from build123d import *

# Parameters (mm, degrees)
F3_W     = 10
F3_H     = 5
F8_DEPTH = 10
F9_T     = -1


with BuildPart() as f6:
    # F6: sweep along a path in F5
    with BuildLine(Plane(origin=(0, 0, 0), x_dir=(0.5735764364, 0.8191520443, 0), z_dir=(0.8191520443, -0.5735764364, 0))) as f6_path:
        Line((-28.3761330307, -7.5), (-32.7062600496, -5))
    # F3 (on line) → F6 (sweep)
    with BuildSketch(Plane(origin=(-18.7595400856, -26.7913997807, 0), x_dir=(-0.8191520443, 0.5735764364, 0), z_dir=(0.5735764364, 0.8191520443, 0))):
        with Locations((0, -5)):
            Rectangle(F3_W, F3_H)
    sweep(path=f6_path.line)

    # F7 (on face) → F8 (cut, through all)
    with BuildSketch(Plane(origin=(4.0957602214, -2.8678821818, 0), x_dir=(0.5735764364, 0.8191520443, 0), z_dir=(0.8191520443, -0.5735764364, 0))):
        Polygon((-28.3761330307, -10), (-28.3761330307, -5), (-30.5411965402, -8.75), align=None)
    extrude(amount=-F8_DEPTH, mode=Mode.SUBTRACT)

    # F9
    f9_openings = [f6.faces().sort_by_distance(p)[0] for p in [
        (-16.896796, -24.131125, -6.875),
        (-18.75954, -26.7914, -5),
    ]]
    offset(amount=F9_T, openings=f9_openings)


solid = f6.part
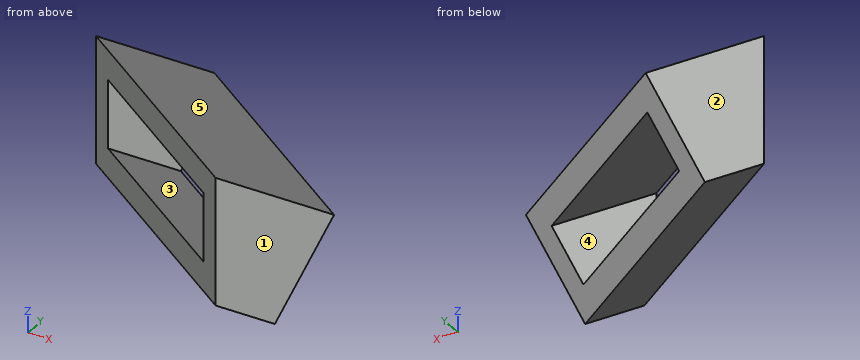
Geometry check sheet. Reference: the model listing, model coordinates, mm. Face numbers are marked on the shaded views. A direction names the side the tool comes from. Give positions to 0.01 mm unless a question says otherwise; leave off trailing zeros. Order: outer loops, then holes, each group sorted by start corner. A loop starts at its lowest first (then second) coordinate and runs counter-clockwise, first axis right, second up. Notation, with made-up numbers: (0, -16) - (29, -16) arc R21 cw to (29, 11) - close; hole circle Ø9 at (-24.75, 3). An arc over 180 degrees is marked (long way). Answer as a JSON object with one key per item and string values.
(1) Cross-section at D-D (y = -28.5). Record the cut outline in (x, z).
Report:
{"outline": "(-16.32, -7.5) - (-13.85, -8.32) - (-13.85, -3.32) - (-16.32, -2.5) - (-16.32, -3.65) - (-15.07, -4.07) - (-15.07, -6.76) - (-16.32, -6.35) - close"}
(2) Depth check by flat-ended pin: pin 1 Ø3 at (x, z) = (-14.5, -6.5) entering from +Y; pin 2 Ø1.5 at (x, y) = (-16, -26.5) entering from -Z; pin 3 Ø1 at (x, y) = (-16.5, -22) entering from -Z. Enter the tip coordinate at first touch or a pass-through.
Report:
{"pin 1": "y = -24.05", "pin 2": "z = -8.75", "pin 3": "through"}
(3) Draft check along Y on the marked faces 1, 2 and 3. Enter one of: released by +Y, released by -Y, zero draft, split by the parting line, or undercut.
Report:
{"face 1": "released by -Y", "face 2": "released by +Y", "face 3": "undercut"}
(4) Material ranges on line 1 (Z direction, x = -18.25, y = -26); line 2 (Z direction, x = -18, y = -25); line 3 (Y direction, x = -20, z = -8), recorded low to high.
Report:
{"line 1": "-8.04 to -6.89, -4.2 to -3.04", "line 2": "-8.6 to -7.44, -4.75 to -3.6", "line 3": "-24.87 to -22.75"}
(5) Cross-section at C-C (z = -5.25). Record the cut outline in (x, y), then the cut area to 3 significant figures.
Report:
{"outline": "(-22.86, -23.92) - (-22.04, -24.5) - (-20.45, -22.23) - (-13.9, -26.82) - (-15.48, -29.09) - (-14.66, -29.66) - (-12.26, -26.23) - (-20.45, -20.49) - close", "area": "19.8 mm^2"}
(6) Tool access check on the marked faces 4 and 5. Record the directions out of +Z, -Z, +X, -X, +Y, -Y that give a thin tool (end or side, any length) a straight path to the whole face; none if there is none.
Report:
{"face 4": "none", "face 5": "+Z, +X, +Y"}
(7) Cross-section at A-A (x = -19). Record the cut outline in (y, z).
Report:
{"outline": "(-26.62, -7.5) - (-23.98, -8.75) - (-23.37, -7.88) - (-26.62, -6.35) - close; (-26.62, -3.65) - (-21.95, -5.87) - (-21.34, -5) - (-26.62, -2.5) - close"}
(8) Cross-section at B-B (y = -25). Record the cut outline in (x, z), then the cut area to 3 significant figures.
Report:
{"outline": "(-21.32, -7.5) - (-17.54, -8.75) - (-16.67, -7.88) - (-21.32, -6.35) - close; (-21.32, -3.65) - (-14.64, -5.87) - (-13.77, -5) - (-21.32, -2.5) - close", "area": "13.1 mm^2"}
